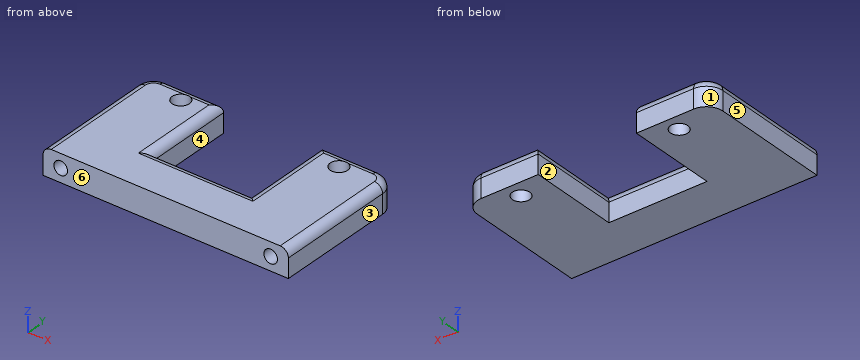
from build123d import *

# Parameters (mm, degrees)
MODEL_R             = 1.6
EXTRUDE_1_DEPTH     = 5
SKETCH_2_R          = 1.25
CUT_EXTRUDE_1_DEPTH = 6
FILLET_1_R          = 1.5


with BuildPart() as part:
    # Model → 凸台-拉伸1 (new body)
    with BuildSketch(Plane.XY):
        with BuildLine():
            Line((241.119901236, 237.095927438), (251.619901236, 237.095927438))
            Line((251.619901236, 237.095927438), (251.619901236, 220.595927438))
            Line((251.619901236, 220.595927438), (269.619901236, 220.595927438))
            Line((269.619901236, 220.595927438), (269.619901236, 237.095927438))
            Line((269.619901236, 237.095927438), (280.119901236, 237.095927438))
            ThreePointArc((280.119901236, 237.095927438), (282.241221579, 236.217247782), (283.119901236, 234.095927438))
            Line((283.119901236, 234.095927438), (283.119901236, 212.095927438))
            Line((283.119901236, 212.095927438), (238.119901236, 212.095927438))
            Line((238.119901236, 212.095927438), (238.119901236, 234.095927438))
            ThreePointArc((238.119901236, 234.095927438), (238.998580892, 236.217247782), (241.119901236, 237.095927438))
        make_face()
        with Locations((246.119901236, 234.095927438)):
            Circle(MODEL_R, mode=Mode.SUBTRACT)
        with Locations((275.119901236, 234.095927438)):
            Circle(MODEL_R, mode=Mode.SUBTRACT)
    extrude(amount=EXTRUDE_1_DEPTH)

    # 草图2 → 切除-拉伸1 (cut)
    with BuildSketch(Plane.XZ.offset(-212.095927438)):
        with Locations(Location((241.369901236, 2.5, 0), (0, 0, 270))):
            Circle(SKETCH_2_R)
        with Locations(Location((279.869901236, 2.5, 0), (0, 0, 270))):
            Circle(SKETCH_2_R)
    extrude(amount=-CUT_EXTRUDE_1_DEPTH, mode=Mode.SUBTRACT)

    # 圆角1
    # the kernel refuses this fillet: 1.5 mm, written as the material it takes off along each edge
    with BuildSketch(Plane(origin=(283.119901236, 234.095927438, 5), x_dir=(0, 0, -1), z_dir=(0, -1, 0))) as fillet_1_piece_1:
        with BuildLine():
            CenterArc((FILLET_1_R, -FILLET_1_R), FILLET_1_R, 90, 90)
            Line((0, -FILLET_1_R), (0, 0))
            Line((0, 0), (FILLET_1_R, 0))
        make_face()
    extrude(amount=25.75, mode=Mode.SUBTRACT)
    with BuildSketch(Plane(origin=(280.119901236, 234.095927438, 5), x_dir=(0, 1, 0), z_dir=(-1, 0, 0))) as fillet_1_piece_2:
        with BuildLine():
            CenterArc((3 - FILLET_1_R, FILLET_1_R), FILLET_1_R, 270, 90)
            Line((3 - FILLET_1_R, 0), (3, 0))
            Line((3, 0), (3, FILLET_1_R))
        make_face()
    revolve(axis=Axis((280.119901236, 234.095927438, 5), (0, 0, -1)), revolution_arc=90, mode=Mode.SUBTRACT)
    with BuildSketch(Plane(origin=(265.869901236, 237.095927438, 5), x_dir=(0, 0, -1), z_dir=(1, 0, 0))) as fillet_1_piece_3:
        with BuildLine():
            CenterArc((FILLET_1_R, -FILLET_1_R), FILLET_1_R, 90, 90)
            Line((0, -FILLET_1_R), (0, 0))
            Line((0, 0), (FILLET_1_R, 0))
        make_face()
    extrude(amount=14.25, mode=Mode.SUBTRACT)
    with BuildSketch(Plane(origin=(269.619901236, 220.595927438, 5), x_dir=(1, 0, 0), z_dir=(0, 1, 0)), Plane(origin=(251.619901236, 240.845927438, 5), x_dir=(-1, 0, 0), z_dir=(0, -1, 0))) as fillet_1_piece_4:
        with BuildLine():
            CenterArc((FILLET_1_R, FILLET_1_R), FILLET_1_R, 180, 90)
            Line((0, FILLET_1_R), (0, 0))
            Line((0, 0), (FILLET_1_R, 0))
        make_face()
    extrude(amount=20.25, mode=Mode.SUBTRACT)
    with BuildSketch(Plane(origin=(251.619901236, 220.595927438, 5), x_dir=(0, -1, 0), z_dir=(1, 0, 0))) as fillet_1_piece_5:
        with BuildLine():
            CenterArc((FILLET_1_R, FILLET_1_R), FILLET_1_R, 180, 90)
            Line((0, FILLET_1_R), (0, 0))
            Line((0, 0), (FILLET_1_R, 0))
        make_face()
    extrude(amount=18, mode=Mode.SUBTRACT)
    with BuildSketch(Plane(origin=(241.119901236, 237.095927438, 5), x_dir=(0, -1, 0), z_dir=(1, 0, 0))) as fillet_1_piece_6:
        with BuildLine():
            CenterArc((FILLET_1_R, FILLET_1_R), FILLET_1_R, 180, 90)
            Line((0, FILLET_1_R), (0, 0))
            Line((0, 0), (FILLET_1_R, 0))
        make_face()
    extrude(amount=14.25, mode=Mode.SUBTRACT)
    with BuildSketch(Plane(origin=(241.119901236, 234.095927438, 5), x_dir=(-1, 0, 0), z_dir=(0, -1, 0))) as fillet_1_piece_7:
        with BuildLine():
            CenterArc((3 - FILLET_1_R, FILLET_1_R), FILLET_1_R, 270, 90)
            Line((3, FILLET_1_R), (3, 0))
            Line((3, 0), (3 - FILLET_1_R, 0))
        make_face()
    revolve(axis=Axis((241.119901236, 234.095927438, 5), (0, 0, -1)), revolution_arc=90, mode=Mode.SUBTRACT)
    with BuildSketch(Plane(origin=(238.119901236, 208.345927438, 5), x_dir=(1, 0, 0), z_dir=(0, 1, 0))) as fillet_1_piece_8:
        with BuildLine():
            CenterArc((FILLET_1_R, FILLET_1_R), FILLET_1_R, 180, 90)
            Line((0, FILLET_1_R), (0, 0))
            Line((0, 0), (FILLET_1_R, 0))
        make_face()
    extrude(amount=25.75, mode=Mode.SUBTRACT)
    with BuildSketch(Plane(origin=(251.619901236, 220.595927438, 5), x_dir=(0, -1, 0), z_dir=(1, 0, 0))) as fillet_1_piece_9a_section:
        with BuildLine():
            CenterArc((FILLET_1_R, FILLET_1_R), FILLET_1_R, 180, 90)
            Line((0, FILLET_1_R), (0, 0))
            Line((0, 0), (FILLET_1_R, 0))
        make_face()
    fillet_1_piece_9a = extrude(amount=21.75, mode=Mode.PRIVATE)
    fillet_1_piece_9a = split(fillet_1_piece_9a, bisect_by=Plane(origin=(269.619901236, 220.256334767, 4.660407329), z_dir=(1, 0, 0)), keep=Keep.TOP, mode=Mode.PRIVATE)
    with BuildSketch(Plane(origin=(269.619901236, 216.845927438, 5), x_dir=(1, 0, 0), z_dir=(0, 1, 0))) as fillet_1_piece_9b_section:
        with BuildLine():
            CenterArc((FILLET_1_R, FILLET_1_R), FILLET_1_R, 180, 90)
            Line((0, FILLET_1_R), (0, 0))
            Line((0, 0), (FILLET_1_R, 0))
        make_face()
    fillet_1_piece_9b = extrude(amount=24, mode=Mode.PRIVATE)
    fillet_1_piece_9b = split(fillet_1_piece_9b, bisect_by=Plane(origin=(269.959493907, 220.595927438, 4.660407329), z_dir=(0, -1, 0)), keep=Keep.TOP, mode=Mode.PRIVATE)
    fillet_1_piece_9 = fillet_1_piece_9a & fillet_1_piece_9b
    add(fillet_1_piece_9, mode=Mode.SUBTRACT)
    with BuildSketch(Plane(origin=(251.619901236, 240.845927438, 5), x_dir=(-1, 0, 0), z_dir=(0, -1, 0))) as fillet_1_piece_10a_section:
        with BuildLine():
            CenterArc((FILLET_1_R, FILLET_1_R), FILLET_1_R, 180, 90)
            Line((0, FILLET_1_R), (0, 0))
            Line((0, 0), (FILLET_1_R, 0))
        make_face()
    fillet_1_piece_10a = extrude(amount=24, mode=Mode.PRIVATE)
    fillet_1_piece_10a = split(fillet_1_piece_10a, bisect_by=Plane(origin=(251.280308564, 220.595927438, 4.660407329), z_dir=(0, -1, 0)), keep=Keep.TOP, mode=Mode.PRIVATE)
    with BuildSketch(Plane(origin=(247.869901236, 220.595927438, 5), x_dir=(0, -1, 0), z_dir=(1, 0, 0))) as fillet_1_piece_10b_section:
        with BuildLine():
            CenterArc((FILLET_1_R, FILLET_1_R), FILLET_1_R, 180, 90)
            Line((0, FILLET_1_R), (0, 0))
            Line((0, 0), (FILLET_1_R, 0))
        make_face()
    fillet_1_piece_10b = extrude(amount=21.75, mode=Mode.PRIVATE)
    fillet_1_piece_10b = split(fillet_1_piece_10b, bisect_by=Plane(origin=(251.619901236, 220.256334767, 4.660407329), z_dir=(-1, 0, 0)), keep=Keep.TOP, mode=Mode.PRIVATE)
    fillet_1_piece_10 = fillet_1_piece_10a & fillet_1_piece_10b
    add(fillet_1_piece_10, mode=Mode.SUBTRACT)


solid = part.part
Geometry: final body of the model. Coordinates: model frame, mm. Face numbers are marked on the shaded views. A direction names the side the tool comes from. Give positions to 0.01 mm unless a question says otherwise; leave off trailing zeros. Write each loop counter-clockwise with the first axis right and the second up, starting at its lowest first coordinate (ties: lowest second). Pieces come first, ordered by that corner, then holes. Notation, with made-up numbers: (47.5, 28) -> (61.5, 28) arc R14 cw to (61.5, 37) -> close; hole circle Ø7 at (-37, 0). An arc over 180 degrees is marked (long way). Answer as a JSON object with one key per item and string values.
1. Ray query, probe 1 along X at (y, z) = (214.9, 2.5); probe 2 along X at (y, z) = (229.75, 1.85); probe 3 along X at (y, z) = (233.5, 4.35). Return the intervals inside material, ascending. Write a range as from..to.
Ans:
{"probe 1": "x = 238.12..240.12, 242.62..278.62, 281.12..283.12", "probe 2": "x = 238.12..251.62, 269.62..283.12", "probe 3": "x = 238.38..244.64, 247.6..251.36, 269.88..273.64, 276.6..282.86"}
2. Cut plane A-A on y = 225.5. Output: boundary loops of the cut face in (x, z).
Ans:
{"outline": "(238.12, 0) -> (251.62, 0) -> (251.62, 3.5) arc R1.5 ccw to (250.12, 5) -> (239.62, 5) arc R1.5 ccw to (238.12, 3.5) -> close; (269.62, 0) -> (283.12, 0) -> (283.12, 3.5) arc R1.5 ccw to (281.62, 5) -> (271.12, 5) arc R1.5 ccw to (269.62, 3.5) -> close"}
3. Mould query, pull axis X, two halves, no side actions, for the marked faces 3, 4, 5 and 6. Classes: pulls with the +X half, pulls with the -X half, needs draft (parallel to the pull), parting line crosses it, or undercut.
Ans:
{"face 3": "pulls with the +X half", "face 4": "undercut", "face 5": "pulls with the -X half", "face 6": "needs draft"}
4. Access query for the marked faces 1 and 2. Directions: +Z, -Z, +X, -X, +Y, -Y. A direction counts if a zero-diameter tool reaches every point of the face in a straight line with its end or side. Return the directions, or none.
Ans:
{"face 1": "+Z, -Z, -X, +Y", "face 2": "+Z, -Z, +Y"}
5. Contact query for flat-ended pins moving along their axis: pin 1 (2 mm diameter, centred on x = 279.87, z = 2.5, fed in from -Y); pin 2 (1.5 mm diameter, centred on x = 260.5, z = 3.5, fed in from +Y); pin 3 (2.5 mm diameter, centred on x = 275.12, y = 234.1, fed in from -Z). Output: stop coordinate, or through.
Ans:
{"pin 1": "stops at y = 218.1", "pin 2": "stops at y = 220.6", "pin 3": "passes through"}
6. Cut plane B-B on z = 2.5. Output: boundary loops of the cut face in (x, y), and give its area (3 significant figures).
Ans:
{"outline": "(238.12, 212.1) -> (240.12, 212.1) -> (240.12, 218.1) -> (242.62, 218.1) -> (242.62, 212.1) -> (278.62, 212.1) -> (278.62, 218.1) -> (281.12, 218.1) -> (281.12, 212.1) -> (283.12, 212.1) -> (283.12, 234.1) arc R3 ccw to (280.12, 237.1) -> (269.62, 237.1) -> (269.62, 220.6) -> (251.62, 220.6) -> (251.62, 237.1) -> (241.12, 237.1) arc R3 ccw to (238.12, 234.1) -> close; hole circle Ø3.2 at (246.12, 234.1); hole circle Ø3.2 at (275.12, 234.1)", "area": "778 mm^2"}
7. Cut plane C-C on x = 259. Output: boundary loops of the cut face in (y, z), and give its area (3 significant figures).
Ans:
{"outline": "(212.1, 0) -> (220.6, 0) -> (220.6, 3.5) arc R1.5 ccw to (219.1, 5) -> (212.1, 5) -> close", "area": "42.0 mm^2"}
